Design review of the part built by this model. Coordinates are the model's own, in mm. Face numbers are marked on the shaded views. A direction names the side the tool comes from. Coordinates: 2 decimals unless noted, no trailing zeros. Write each loop counter-clockwise with the first axis right and the second up, starting at its lowest first coordinate (ties: lowest second). Pieces come first, ordered by that corner, then holes. Notation, with made-up numbers: (66, 16.25) - (118, 16.25) arc R18 ccw to (118, 50.25) - close; hole circle Ø3 at (-3, -23). An arc over 180 degrees is marked (long way). One line per item, written item: value.
from build123d import *

# Parameters (mm, degrees)
F0_R        = 56.6549127416
F1_DEPTH    = 10
F2_W        = 43.7059700489
F2_H        = 56.300342083
F3_DEPTH    = 25
F4_T4_DEPTH = 210.6013213609


# Not quite as in the source:
# - a fillet or chamfer that OpenCascade refuses, or shapes differently, is made with other operations: its cross-section is extruded or revolved along the edge and cut away or added


with BuildPart() as f1:
    # F0 (on Top) → F1 (new body)
    with BuildSketch(Plane.XY):
        Circle(F0_R)
    extrude(amount=F1_DEPTH)

    # F2 (on face) → F3 (join)
    with BuildSketch(Plane.XY.offset(10)):
        Rectangle(F2_W, F2_H)
    extrude(amount=F3_DEPTH)

    # F4: chamfer of 30 on 1 edges, made by hand


with BuildPart() as f4_tool2:
    # F4_s3 → F4_t4 (new body)
    with BuildSketch(Plane.XZ.offset(-105.3006606805)):
        Polygon((-21.8529850245, 5), (8.1470149755, 35), (-21.8529850245, 35), align=None)
    extrude(amount=F4_T4_DEPTH)

    split(bisect_by=Plane.XY.offset(10), keep=Keep.TOP)


with BuildPart() as f1_1:
    add(f1.part)

    # F4_t1: cut F4_tool2
    add(f4_tool2.part, mode=Mode.SUBTRACT)


solid = f1_1.part
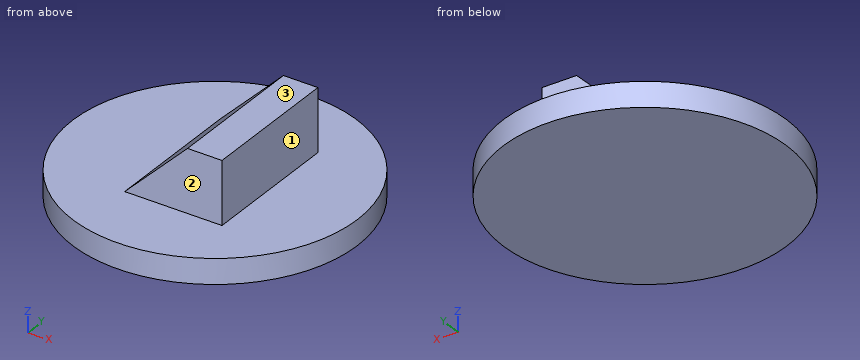
1. Consider section C-C, the plane x = 0. Write out the cut boundary in (y, z), then the cut area to 3 significant figures.
Answer block:
outline: (-56.65, 0) - (56.65, 0) - (56.65, 10) - (28.15, 10) - (28.15, 26.85) - (-28.15, 26.85) - (-28.15, 10) - (-56.65, 10) - close
area: 2,080 mm^2
2. For the marked faces 1, 2 and 3, list the 3-axis set-ups (+Z, -Z, +X, -X, +Y, -Y) from which the entire face can be reached by the end or side of a thin tool; tool diameter is ignored.
Answer block:
face 1: +Z, +X, +Y, -Y
face 2: +Z, +X, -X, -Y
face 3: +Z, +X, -X, +Y, -Y
3. Consider section A-A, the plane y = 0. Write out the cut boundary in (x, z).
Answer block:
outline: (-56.65, 0) - (56.65, 0) - (56.65, 10) - (21.85, 10) - (21.85, 35) - (8.15, 35) - (-16.85, 10) - (-56.65, 10) - close
4. Wall thickness on line 1 along Z through (x, y) = (-13, 43); line 2 along X through (y, z) = (-6, 22); line 3 along X through (y, z) = (10, 9): over which ranges is each line inside the solid? List them lowest first.
Answer block:
line 1: z = 0 to 10
line 2: x = -4.85 to 21.85
line 3: x = -55.77 to 55.77
5. Consider section B-B, the plane z = 4. Write out the cut boundary in (x, y).
Answer block:
outline: circle Ø113.31 at (0, 0)
6. Insertion check: pin 1 Ø8 at (y, z) = (-4.5, 30.5) entering from +X; pin 2 Ø7.5 at (x, z) = (-2.5, 16.5) entering from -Y; pin 3 Ø7.5 at (x, z) = (8.5, 23) entering from +Y. Each pin has a flat end and moves straight along its axis. Give the tip position at first contact, or say it passes through.
Answer block:
pin 1: stops at x = 21.85
pin 2: stops at y = -28.15
pin 3: stops at y = 28.15
7. Consider section D-D, the plane y = 43.5. Write out the cut boundary in (x, z), then the cut area to 3 significant figures.
Answer block:
outline: (-36.3, 0) - (36.3, 0) - (36.3, 10) - (-36.3, 10) - close
area: 726 mm^2
